```python
from build123d import *

# Parameters (mm, degrees)
SKETCH2_W           = 10
SKETCH2_H           = 12
BOSS_EXTRUDE1_DEPTH = 10
SKETCH3_R           = 1.925
CUT_EXTRUDE1_DEPTH  = 4.5
SKETCH4_R           = 1.925
CUT_EXTRUDE2_DEPTH  = 10


with BuildPart() as part:
    # Sketch2 → Boss-Extrude1 (new body)
    with BuildSketch(Plane(origin=(0, 0, 0), x_dir=(1, 0, 0), z_dir=(0, 1, 0))):
        with Locations((-18.157041848, 40.649833306)):
            Rectangle(SKETCH2_W, SKETCH2_H)
    extrude(amount=BOSS_EXTRUDE1_DEPTH)

    # Sketch3 → Cut-Extrude1 (cut)
    with BuildSketch(Plane.XY.offset(-34.649833306)):
        with Locations((-18.157041848, 5)):
            Circle(SKETCH3_R)
    extrude(amount=-CUT_EXTRUDE1_DEPTH, mode=Mode.SUBTRACT)

    # Sketch4 → Cut-Extrude2 (cut)
    with BuildSketch(Plane(origin=(-13.157041848, 0, 0), x_dir=(0, 0, -1), z_dir=(1, 0, 0))):
        with Locations((42.649833306, 5)):
            Circle(SKETCH4_R)
    extrude(amount=-CUT_EXTRUDE2_DEPTH, mode=Mode.SUBTRACT)


solid = part.part
```
Can you work these out from the model? Positions are in its coordinate system, mm. A direction names the side the tool comes from. Round coordinates to 2 decimals unless told otherwise and drop trailing zeros. Loops run counter-clockwise (first coordinate to the right, second up) from the corner with the lowest first, then second, coordinate; pieces in that order, holes last. Notation, with made-up numbers: M -11,-22.5 L 6,-22.5 A12 cw 6,-3.5 Z; hole C -2.5,32 d5. An arc over 180 degrees is marked long. Answer as a JSON object with one key per item and string values. Group by question number.
Q1. Will these pins go through, and if not, where does the flat tip stop? pin 1 (3.5 mm diameter, centred on y = 5, z = -42.65, fed in from +X); pin 2 (2.5 mm diameter, centred on x = -18.16, y = 5, fed in from +Z).
Q2. We'd pull the mould along Y, two halves only. Please class faces 3 (the flat face through (-18, 0, -41)), 4 (the cylindrical face through (-18.087, 5.085, -40.727)), 5 (the flat face through (-13.157, 4.93, -40.57)): +Y half, -Y half, draft (parallel to the pull), parting line (faces both ways), or undercut.
Q3. Imagine slicing it at A-A, the plane y = 5. Please give me the cut outline in (x, z), then the cut area to 3 significant figures.
Q4. Please list where these lines run through material, in increasing order: L1, parallel to Y at x = -18.5, z = -42.5; L2, parallel to Y at x = -18.25, z = -44; L3, parallel to X at y = 6, z = -38.
Q5. Imagine slicing it at C-C, the plane z = -42.75. Please give me the cut outline in (x, y), then the cut area to 3 significant figures.
Q6. Imagine slicing it at B-B, the plane x = -20.5. Please give me the cut outline in (y, z) (3 decimals), then the cut area to 3 significant figures.
Q7. Imagine slicing it at D-D, the plane y = 6.75. Please give me the cut outline in (x, z), then the cut area to 3 significant figures.
Q8. On a 3-axis mill with a long thin cutter (end or side, diameter ignored), from which of +Z, -Z, +X, -X, +Y, -Y can I reach the whole of each face in a straight line? I mean faces 1 (the flat face through (-18, 5, -39.15)), 2 (the flat face through (-18, 5, -46.65)). Say none if no direction works.
Findings:
{
 "1": {"pin 1": "passes through", "pin 2": "stops at z = -39.15"},
 "2": {"face 3": "-Y half", "face 4": "undercut", "face 5": "draft"},
 "3": {"outline": "M -23.16,-46.65 L -13.16,-46.65 L -13.16,-44.57 L -23.16,-44.57 Z; M -23.16,-40.72 L -13.16,-40.72 L -13.16,-34.65 L -16.23,-34.65 L -16.23,-39.15 L -20.08,-39.15 L -20.08,-34.65 L -23.16,-34.65 Z", "area": "64.2 mm2"},
 "4": {"L1": "y = 0 to 3.08, 6.92 to 10", "L2": "y = 0 to 3.63, 6.37 to 10", "L3": "x = -23.16 to -19.8, -16.51 to -13.16"},
 "5": {"outline": "M -23.16,0 L -13.16,0 L -13.16,3.08 L -23.16,3.08 Z; M -23.16,6.92 L -13.16,6.92 L -13.16,10 L -23.16,10 Z", "area": "61.6 mm2"},
 "6": {"outline": "M 0,-46.65 L 10,-46.65 L 10,-34.65 L 0,-34.65 Z; hole C 5,-42.65 d3.85", "area": "108 mm2"},
 "7": {"outline": "M -23.16,-46.65 L -13.16,-46.65 L -13.16,-43.45 L -23.16,-43.45 Z; M -23.16,-41.85 L -13.16,-41.85 L -13.16,-34.65 L -17.36,-34.65 L -17.36,-39.15 L -18.96,-39.15 L -18.96,-34.65 L -23.16,-34.65 Z", "area": "96.7 mm2"},
 "8": {"face 1": "+Z", "face 2": "-Z, +X, -X, +Y, -Y"}
}
